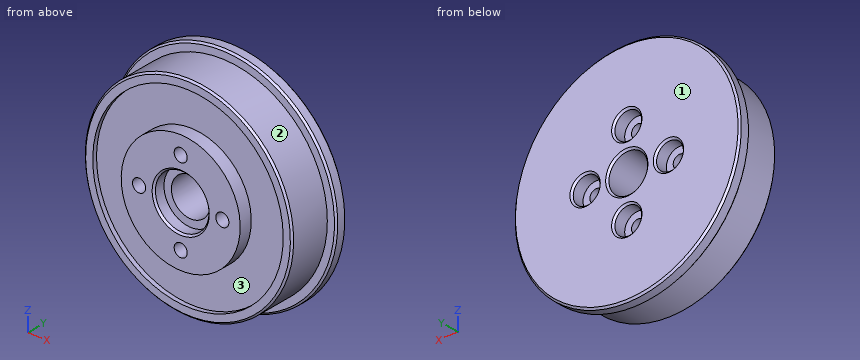
from build123d import *

# Parameters (mm, degrees)
SKETCH_1_R          = 19
EXTRUDE_1_DEPTH     = 10.45
SKETCH_2_R          = 35.878367213
SKETCH_2_R_2        = 17.5
SKETCH_2_R_3        = 10
CUT_EXTRUDE_1_DEPTH = 1.45
SKETCH_2_3_R        = 35.878367213
SKETCH_2_3_R_2      = 17.5
CUT_EXTRUDE_2_DEPTH = 8.45
SKETCH_3_R          = 3.25
SKETCH_3_R_2        = 1.1
CUT_EXTRUDE_3_DEPTH = 29.83058272
CUT_EXTRUDE_START   = 8.2
SKETCH_3_3_R        = 2.25
CUT_EXTRUDE_4_DEPTH = 21.63058272
SKETCH_4_R          = 16
SKETCH_4_R_2        = 10
CUT_EXTRUDE_5_DEPTH = 2.2
SKETCH_5_R          = 4.5
CUT_EXTRUDE_6_DEPTH = 2
CHAMFER_1_SIZE      = 0.3


with BuildPart() as part:
    # Sketch 1 → Extrude 1 (new body)
    with BuildSketch(Plane(origin=(0, 0, 0), x_dir=(1, 0, 0), z_dir=(0, 1, 0))):
        with Locations(Location((0, 0, 0), (0, 0, 270))):
            Circle(SKETCH_1_R)
    extrude(amount=EXTRUDE_1_DEPTH)

    # Sketch 2 → Cut-Extrude 1 (cut)
    # profile 1 of 2: a face of its own
    with BuildSketch(Plane(origin=(0, 0, 0), x_dir=(1, 0, 0), z_dir=(0, 1, 0))):
        Circle(SKETCH_2_R)
        Circle(SKETCH_2_R_2, mode=Mode.SUBTRACT)
    # profile 2 of 2: a face of its own
    with BuildSketch(Plane(origin=(0, 0, 0), x_dir=(1, 0, 0), z_dir=(0, 1, 0))):
        Circle(SKETCH_2_R_2)
        with Locations(Location((0, 0, 0), (0, 0, 270))):
            Circle(SKETCH_2_R_3, mode=Mode.SUBTRACT)
    extrude(amount=CUT_EXTRUDE_1_DEPTH, mode=Mode.SUBTRACT)

    # Sketch 2_3 → Cut-Extrude 2 (cut)
    with BuildSketch(Plane(origin=(0, 0, 0), x_dir=(1, 0, 0), z_dir=(0, 1, 0))):
        Circle(SKETCH_2_3_R)
        with Locations(Location((0, 0, 0), (0, 0, 270))):
            Circle(SKETCH_2_3_R_2, mode=Mode.SUBTRACT)
    extrude(amount=CUT_EXTRUDE_2_DEPTH, mode=Mode.SUBTRACT)

    # Sketch 3 → Cut-Extrude 3 (cut, through all)
    with BuildSketch(Plane(origin=(0, 0, 0), x_dir=(1, 0, 0), z_dir=(0, 1, 0))):
        with Locations(Location((0, 0, 0), (0, 0, 270))):
            Circle(SKETCH_3_R)
        with Locations(Location((0, 7, 0), (0, 0, 270))):
            Circle(SKETCH_3_R_2)
        with Locations(Location((-7, 0, 0), (0, 0, 270))):
            Circle(SKETCH_3_R_2)
        with Locations(Location((0, -7, 0), (0, 0, 270))):
            Circle(SKETCH_3_R_2)
        with Locations(Location((7, 0, 0), (0, 0, 270))):
            Circle(SKETCH_3_R_2)
    extrude(amount=CUT_EXTRUDE_3_DEPTH, mode=Mode.SUBTRACT)

    # Sketch 3_3 → Cut-Extrude 4 (cut, through all)
    with BuildSketch(Plane(origin=(0, 0, 0), x_dir=(1, 0, 0), z_dir=(0, 1, 0)).offset(CUT_EXTRUDE_START)):
        with Locations(Location((0, 7, 0), (0, 0, 270))):
            Circle(SKETCH_3_3_R)
        with Locations(Location((7, 0, 0), (0, 0, 270))):
            Circle(SKETCH_3_3_R)
        with Locations(Location((0, -7, 0), (0, 0, 270))):
            Circle(SKETCH_3_3_R)
        with Locations(Location((-7, 0, 0), (0, 0, 270))):
            Circle(SKETCH_3_3_R)
    extrude(amount=CUT_EXTRUDE_4_DEPTH, mode=Mode.SUBTRACT)

    # Sketch 4 → Cut-Extrude 5 (cut)
    with BuildSketch(Plane(origin=(0, 0, 0), x_dir=(1, 0, 0), z_dir=(0, 1, 0))):
        with Locations(Location((0, 0, 0), (0, 0, 270))):
            Circle(SKETCH_4_R)
        with Locations(Location((0, 0, 0), (0, 0, 270))):
            Circle(SKETCH_4_R_2, mode=Mode.SUBTRACT)
    extrude(amount=CUT_EXTRUDE_5_DEPTH, mode=Mode.SUBTRACT)

    # Sketch 5 → Cut-Extrude 6 (cut)
    with BuildSketch(Plane(origin=(0, 0, 0), x_dir=(1, 0, 0), z_dir=(0, 1, 0))):
        with Locations(Location((0, 0, 0), (0, 0, 270))):
            Circle(SKETCH_5_R)
    extrude(amount=CUT_EXTRUDE_6_DEPTH, mode=Mode.SUBTRACT)

    # Chamfer 1
    chamfer_1_edges = [part.edges().sort_by_distance(p)[0] for p in [
        (0, 8.45, -19),
        (0, 1.45, -17.5),
        (0, 10.45, -3.25),
        (0, 10.45, -19),
        (-7, 10.45, -2.25),
        (0, 10.45, -9.25),
        (7, 10.45, -2.25),
        (0, 10.45, 4.75),
        (0, 0, -4.5),
    ]]
    chamfer(chamfer_1_edges, length=CHAMFER_1_SIZE)


solid = part.part
The model under review builds one solid part; all positions refer to its coordinate system, in mm. Face numbers are marked on the shaded views. Coordinates: 2 decimals unless noted, no trailing zeros. Write each loop counter-clockwise with the first axis right and the second up, starting at its lowest first coordinate (ties: lowest second). Pieces come first, ordered by that corner, then holes. Notation, with made-up numbers: M 26.5,50 L 41.5,50 A15 ccw 41.5,73 Z; hole C 19.5,81 d1. An arc over 180 degrees is marked long. Put each result on its own line as item: value.
1) Add section A-A on y = 4.75. Give the boundary of the cut face in (x, z), then the cut area to 3 significant figures.
Computed:
outline: C 0,0 d35; hole C -7,0 d2.2; hole C 0,0 d6.5; hole C 0,-7 d2.2; hole C 0,7 d2.2; hole C 7,0 d2.2
area: 914 mm2
2) Draft analysis for pull direction X (two halves, no side actions). For the marked faces 1, 2 and 3, state which applies: released by +X, released by -X, zero draft, split by the parting line, or undercut.
Computed:
face 1: zero draft
face 2: split by the parting line
face 3: undercut
3) Add section B-B on x = 0. State how many separate pieces and enclosed holes the cut face has, then the cut area to 3 significant figures.
Computed:
separate pieces: 4
enclosed holes: 0
area: 211 mm2
4) Clearance check with flat-ended pins moving along their axes: pin 1 Ø3 at (x, y) = (0, 3.5) entering from +Z; pin 2 Ø4 at (x, y) = (6, 9) entering from +Z; pin 3 Ø3.5 at (x, z) = (-7, 0) entering from +Y. State where each tip first meets the part, or that it passes through.
Computed:
pin 1: stops at z = 17.5
pin 2: stops at z = 18.57
pin 3: stops at y = 8.2
5) Wall thickness on probe 1 along X at (y, z) = (1.75, 0); probe 2 along X at (y, z) = (6.75, 0); probe 3 along Z at (x, y) = (0, 9.1): over which ranges is each line inside the solid? List them lowest first. Write a range as [from, to].
Computed:
probe 1: x = [-17.5, -16], [-10, -8.1], [-5.9, -4.5], [4.5, 5.9], [8.1, 10], [16, 17.5]
probe 2: x = [-17.5, -8.1], [-5.9, -3.25], [3.25, 5.9], [8.1, 17.5]
probe 3: z = [-19, -9.25], [-4.75, -3.25], [3.25, 4.75], [9.25, 19]
